from build123d import *

# Parameters (mm, degrees)
SKETCH1_W                                         = 173.0375
SKETCH1_H                                         = 36.27882
EXTRUDE2_DEPTH                                    = 6.35
SKETCH8_W                                         = 6.35
SKETCH8_H                                         = 36.27882
EXTRUDE7_DEPTH                                    = 3.175
EXTRUDE8_DEPTH                                    = 89.627618702
SKETCH19_R                                        = 3.96875
EXTRUDE9_DEPTH                                    = 89.627618702
CSK_FOR_3_FLAT_HEAD_SOCKET_CAP_SCREW1_D           = 2.794
CSK_FOR_3_FLAT_HEAD_SOCKET_CAP_SCREW1_CSINK_D     = 5.51688
CSK_FOR_3_FLAT_HEAD_SOCKET_CAP_SCREW1_CSINK_ANGLE = 82
CSK_FOR_3_FLAT_HEAD_SOCKET_CAP_SCREW2_D           = 2.794
CSK_FOR_3_FLAT_HEAD_SOCKET_CAP_SCREW2_CSINK_D     = 5.51688
CSK_FOR_3_FLAT_HEAD_SOCKET_CAP_SCREW2_CSINK_ANGLE = 82


with BuildPart() as part:
    # Sketch1 → Extrude2 (new body)
    with BuildSketch(Plane.XY):
        Rectangle(SKETCH1_W, SKETCH1_H)
    extrude(amount=EXTRUDE2_DEPTH)

    # Sketch8 → Extrude7 (cut)
    with BuildSketch(Plane.XY.offset(6.35)):
        with Locations((-83.34375, 0)):
            Rectangle(SKETCH8_W, SKETCH8_H)
        with Locations((65.20561, 0)):
            Rectangle(SKETCH8_W, SKETCH8_H)
    extrude(amount=-EXTRUDE7_DEPTH, mode=Mode.SUBTRACT)

    # Sketch18 → Extrude8 (cut, through all)
    with BuildSketch(Plane.XY.offset(6.35)):
        Polygon((86.51875, 0), (68.38061, 18.13941), (113.519162523, 18.13941), (113.519162523, -18.13941), (68.38061, -18.13941), align=None)
    extrude(amount=-EXTRUDE8_DEPTH, mode=Mode.SUBTRACT)

    # Sketch19 → Extrude9 (cut, through all)
    with BuildSketch(Plane.XY.offset(6.35)):
        with Locations((-0.79375, 0)):
            Circle(SKETCH19_R)
    extrude(amount=-EXTRUDE9_DEPTH, mode=Mode.SUBTRACT)

    # CSK for #3 Flat Head Socket Cap Screw1 (through all)
    with Locations(Plane(origin=(2.381898793, -14.071004552, 0), x_dir=(-1, 0, 0), z_dir=(0, 0, -1))):
        with Locations((-62.823711207, 25.860414552), (-62.823711207, 0.892214552)):
            CounterSinkHole(CSK_FOR_3_FLAT_HEAD_SOCKET_CAP_SCREW1_D / 2, CSK_FOR_3_FLAT_HEAD_SOCKET_CAP_SCREW1_CSINK_D / 2, counter_sink_angle=CSK_FOR_3_FLAT_HEAD_SOCKET_CAP_SCREW1_CSINK_ANGLE)

    # CSK for #3 Flat Head Socket Cap Screw2 (through all)
    with Locations(Plane(origin=(2.381898793, -14.071004552, 0), x_dir=(-1, 0, 0), z_dir=(0, 0, -1))):
        with Locations((85.725648793, 25.860414552), (85.725648793, 0.892214552)):
            CounterSinkHole(CSK_FOR_3_FLAT_HEAD_SOCKET_CAP_SCREW2_D / 2, CSK_FOR_3_FLAT_HEAD_SOCKET_CAP_SCREW2_CSINK_D / 2, counter_sink_angle=CSK_FOR_3_FLAT_HEAD_SOCKET_CAP_SCREW2_CSINK_ANGLE)


solid = part.part
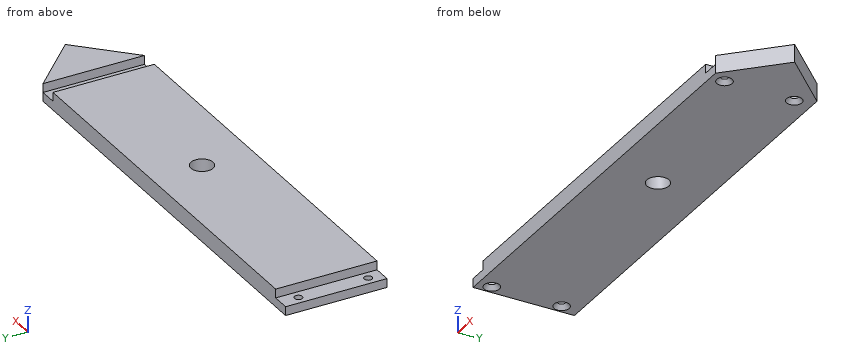
For this review, take the finished solid that the model builds, in its own axes (mm). Round coordinates to 2 decimals unless told otherwise and drop trailing zeros. Loops run counter-clockwise (first coordinate to the right, second up) from the corner with the lowest first, then second, coordinate; pieces in that order, holes last. Notation, with made-up numbers: (-4, -22) - (42, -22) arc R22 ccw to (42, 6) - close; hole circle Ø9 at (-13, 3). An arc over 180 degrees is marked (long way). Answer as CSV lines item,"result".
(1) Consider section C-C on y = -7.5. Give the boundary of the cut face in (x, z) (3 decimals).
Checked values:
outline,"(-86.519, 0) - (79.019, 0) - (79.019, 6.35) - (68.381, 6.35) - (68.381, 3.175) - (62.031, 3.175) - (62.031, 6.35) - (-80.169, 6.35) - (-80.169, 3.175) - (-86.519, 3.175) - close"
(2) Consider section A-A on z = 4.5. Give the boundary of the cut face in (x, y) (1 decimal).
Checked values:
outline,"(-80.2, -18.1) - (62, -18.1) - (62, 18.1) - (-80.2, 18.1) - close; (68.4, -18.1) - (86.5, 0) - (68.4, 18.1) - close; hole circle Ø7.9 at (-0.8, 0)"
(3) Wall thickness on line 1 (X direction, y = -13.5, z = 2.25); line 2 (X direction, y = -1, z = 4.5); line 3 (X direction, y = 10.5, z = 3.75): over which ranges is each line inside the solid? List them lowest first.
Checked values:
line 1,"x = -86.52 to -84.7, -81.98 to 63.85, 66.57 to 73.02"
line 2,"x = -80.17 to -4.63, 3.05 to 62.03, 68.38 to 85.52"
line 3,"x = -80.17 to 62.03, 68.38 to 76.02"
(4) Consider section B-B on y = 16. Give the boundary of the cut face in (x, z) (3 decimals), then the cut area to 3 significant figures.
Checked values:
outline,"(-86.519, 0) - (70.52, 0) - (70.52, 6.35) - (68.381, 6.35) - (68.381, 3.175) - (62.031, 3.175) - (62.031, 6.35) - (-80.169, 6.35) - (-80.169, 3.175) - (-86.519, 3.175) - close"
area,"957 mm2"
(5) Insertion check: P1, Ø1.9, axis at x = 66, y = -6, coming from the +Z side (3 decimals); P2, Ø4.5, axis at x = -83.34, y = 11.79, coming from the -Z side; P3, Ø2.5, axis at y = -6, z = 4.5, coming from the -X side; P4, Ø12.5, axis at x = -0.79, y = 0, coming from the -Z side. Each pin has a flat end and moves straight along its axis. Give the tip position at first contact, or say it passes through.
Checked values:
P1,"stops at z = 3.175"
P2,"stops at z = 0.58"
P3,"stops at x = -80.17"
P4,"stops at z = 0"
